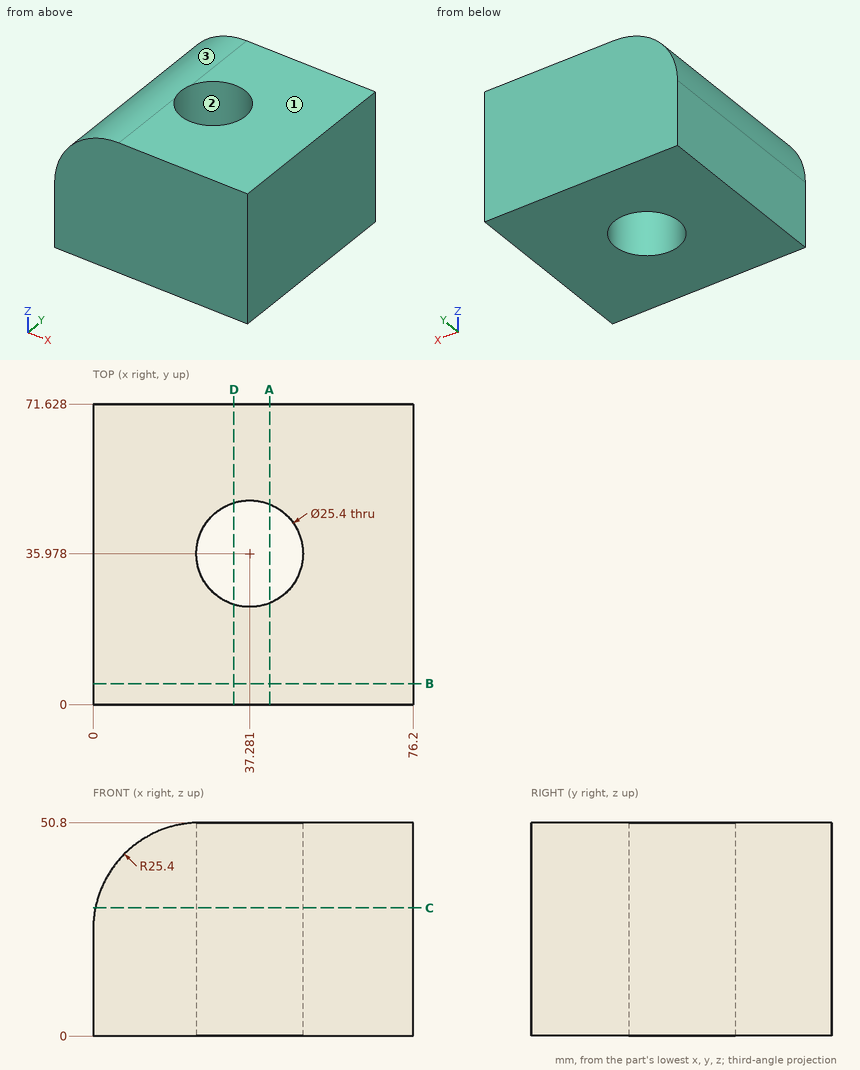
For this review, use the dimensioned drawing (mm, ordinates from the lowest corner) and the shaded views. Coordinates: 2 decimals unless noted, no trailing zeros. Loops run counter-clockwise (first coordinate to the right, second up) from the corner with the lowest first, then second, coordinate; pieces in that order, holes last. Notation, with made-up numbers: (43, -1.5) -> (85, -1.5) arc R26 ccw to (85, 37.5) -> close; hole circle Ø4 at (63.25, -37.5). An arc over 180 degrees is marked (long way). Use a Markdown table: item, result. Add a question column.
Item 1: We need section A-A, the plane x = 42. Write out the cut boundary in (y, z).
Item 2: The part is to be moulded in two halves that separate along X. For the marked faces 1, 2 and 3, say which applies: +X half, -X half, draft (parallel to the pull), parting line (faces both ways), or undercut.
Item 3: We need section D-D, the plane x = 33.5. Write out the cut boundary in (y, z).
Item 4: We need section B-B, the plane y = 5. Write out the cut boundary in (x, z).
Item 5: We need section C-C, the plane z = 30.5. Write out the cut boundary in (x, y), and give its area (3 significant figures).
Item 6: Clearance check with flat-ended pins moving along their axes: P1, Ø5, axis at x = 21, y = 32, coming from the +Z side; P2, Ø3, axis at y = 19.5, z = 37, coming from the -X side; P3, Ø6, axis at x = 10, y = 39.5, coming from the +Z side. State where each tip first meets the part, or that it passes through.
Item 7: Wall thickness on L1, parallel to Y at x = 31.5, z = 7 (1 decimal); L2, parallel to X at y = 41.5, z = 42.5 (1 decimal); L3, parallel to X at y = 36.5, z = 46: over which ranges is each line inside the solid? List them lowest first. Write a range as from..to.
Numbers:
| question | item | result |
|---|---|---|
| 1 | outline | (0, 0) -> (24.19, 0) -> (24.19, 50.8) -> (0, 50.8) -> close; (47.77, 0) -> (71.63, 0) -> (71.63, 50.8) -> (47.77, 50.8) -> close |
| 2 | face 1 | draft |
| 2 | face 2 | undercut |
| 2 | face 3 | -X half |
| 3 | outline | (0, 0) -> (23.85, 0) -> (23.85, 50.8) -> (0, 50.8) -> close; (48.1, 0) -> (71.63, 0) -> (71.63, 50.8) -> (48.1, 50.8) -> close |
| 4 | outline | (0, 0) -> (76.2, 0) -> (76.2, 50.8) -> (25.4, 50.8) arc R25.4 ccw to (0, 25.4) -> close |
| 5 | outline | (0.52, 0) -> (76.2, 0) -> (76.2, 71.63) -> (0.52, 71.63) -> close; hole circle Ø25.4 at (37.28, 35.98) |
| 5 | area | 4,910 mm^2 |
| 6 | P1 | stops at z = 50.73 |
| 6 | P2 | stops at x = 2.09 |
| 6 | P3 | stops at z = 47.57 |
| 7 | L1 | y = 0..24.7, 47.3..71.6 |
| 7 | L2 | x = 6.6..25.8, 48.7..76.2 |
| 7 | L3 | x = 10.54..24.59, 49.97..76.2 |
